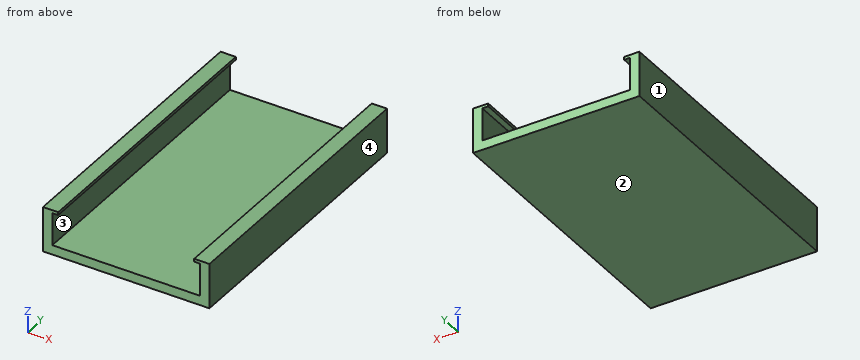
Autodesk Inventor part; units mm, degrees
ref_plane "YZ Plane" through (0, 0, 0) normal (1, 0, 0) x (0, 1, 0)
ref_plane "XZ Plane" through (0, 0, 0) normal (0, 1, 0) x (-1, 0, 0)
ref_plane "XY Plane" through (0, 0, 0) normal (0, 0, 1) x (1, 0, 0)
sketch "Sketch1" plane through (0, 0, 0) normal (0, 0, 1) x (1, 0, 0)
  line L0 (-9.7052, 150.741) -> (79.6698, 150.741)
  line L1 (79.6698, 150.741) -> (79.6698, -1.659)
  line L2 (79.6698, -1.659) -> (-9.7052, -1.659)
  line L3 (-9.7052, -1.659) -> (-9.7052, 150.741)
  point P0 (0, 0)
  dimension "d0" = 89.375
  dimension "d1" = 152.4
extrude "Extrusion1" add sketch "Sketch1" along normal blind 5.08
sketch "Sketch2" plane through (0, 0, 5.08) normal (0, 0, 1) x (1, 0, 0)
  line L0 (79.6698, 150.741) -> (-9.7052, 150.741)
  line L1 (-9.7052, -1.659) -> (79.6698, -1.659)
  line L2 (-9.7052, 150.741) -> (-4.7052, 150.741)
  line L3 (-4.7052, 150.741) -> (-4.7052, -1.659)
  line L4 (-4.7052, -1.659) -> (-9.7052, -1.659)
  line L5 (-9.7052, -1.659) -> (-9.7052, 150.741)
  line L6 (79.6698, 150.741) -> (74.6698, 150.741)
  line L7 (74.6698, 150.741) -> (74.6698, -1.659)
  line L8 (74.6698, -1.659) -> (79.6698, -1.659)
  line L9 (79.6698, -1.659) -> (79.6698, 150.741)
  point P0 (0, 0)
  dimension "d4" = 5
  dimension "d5" = 5
extrude "Extrusion2" add sketch "Sketch2" along normal blind 19.05 contours L9 L1 L7 L0 | L3 L1 L5 L0
sketch "Sketch3" plane through (-4.7052, -1.659, 5.08) normal (1, 0, 0) x (0, 0, -1)
  line L0 (0, 152.4) -> (-19.05, 152.4)
  line L1 (0, 0) -> (-19.05, 0)
  line L2 (-19.05, 152.4) -> (-17.4625, 152.4)
  line L3 (-17.4625, 152.4) -> (-17.4625, 0)
  line L4 (-17.4625, 0) -> (-19.05, 0)
  line L5 (-19.05, 0) -> (-19.05, 152.4)
  point P0 (5.08, 1.659)
  dimension "d8" = 1.5875
sketch "Sketch4" plane through (74.6698, -1.659, 5.08) normal (-1, 0, 0) x (0, 0, 1)
  line L0 (19.05, 152.4) -> (19.05, 0)
  line L1 (0, 0) -> (19.05, 0)
  line L2 (19.05, 152.4) -> (17.4625, 152.4)
  line L3 (17.4625, 152.4) -> (17.4625, 0)
  line L4 (17.4625, 0) -> (19.05, 0)
  line L5 (19.05, 0) -> (19.05, 152.4)
  point P0 (-5.08, 1.659)
  dimension "d9" = 1.5875
extrude "Extrusion3" add sketch "Sketch4" along normal blind 3.175
extrude "Extrusion4" add sketch "Sketch3" along normal blind 3.175
properties part number "Phone Mount"
Check sheet for the modelled part. Datum: model origin and axes. Units: mm. Face numbers are marked on the shaded views. Give positions to 0.01 mm unless a question says otherwise; leave off trailing zeros. Order: outer loops, then holes, each group sorted by start corner. A loop starts at its lowest first (then second) coordinate and runs counter-clockwise, first axis right, second up. Notation, with made-up numbers: (-16, -2) -> (19, -2) arc R9 ccw to (19, 11) -> close; hole circle Ø10 at (16, -40). An arc over 180 degrees is marked (long way). Return JSON: item names as keys, results as strings.
1. Material ranges on probe 1 along X at (y, z) = (67, 20); probe 2 along Z at (x, y) = (69, 39), recorded low to high. Write a range as [from, to].
From the geometry:
{"probe 1": "[-9.71, -4.71], [74.67, 79.67]", "probe 2": "[0, 5.08]"}
2. Mould release check, pull along X, two halves, no side actions. Record for the marked faces 1, 2, 3 and 4: +X half, -X half, draft (parallel to the pull), parting line (faces both ways), or undercut.
From the geometry:
{"face 1": "-X half", "face 2": "draft", "face 3": "undercut", "face 4": "+X half"}
3. Cross-section at C-C, the plane y = 74. Record the cut outline in (x, z), plus the area to 3 significant figures.
From the geometry:
{"outline": "(-9.71, 0) -> (79.67, 0) -> (79.67, 24.13) -> (71.49, 24.13) -> (71.49, 22.54) -> (74.67, 22.54) -> (74.67, 5.08) -> (-4.71, 5.08) -> (-4.71, 22.54) -> (-1.53, 22.54) -> (-1.53, 24.13) -> (-9.71, 24.13) -> close", "area": "655 mm^2"}
4. Cross-section at D-D, the plane x = 66. Record the cut outline in (y, z), plus the area to 3 significant figures.
From the geometry:
{"outline": "(-1.66, 0) -> (150.74, 0) -> (150.74, 5.08) -> (-1.66, 5.08) -> close", "area": "774 mm^2"}
5. Cross-section at A-A, the plane z = 15. Record the cut outline in (x, y).
From the geometry:
{"outline": "(-9.71, -1.66) -> (-4.71, -1.66) -> (-4.71, 150.74) -> (-9.71, 150.74) -> close; (74.67, -1.66) -> (79.67, -1.66) -> (79.67, 150.74) -> (74.67, 150.74) -> close"}
6. Cross-section at B-B, the plane x = -3. Record the cut outline in (y, z).
From the geometry:
{"outline": "(-1.66, 0) -> (150.74, 0) -> (150.74, 5.08) -> (-1.66, 5.08) -> close; (-1.66, 22.54) -> (150.74, 22.54) -> (150.74, 24.13) -> (-1.66, 24.13) -> close"}
7. Go/stop test with a flat-tipped pin: P1, Ø1.5, axis at x = 44.5, y = 103, coming from the +Z side. Record where the tip stops, or that it passes through.
From the geometry:
{"P1": "z = 5.08"}
